from build123d import *

# Parameters (mm, degrees)
SKETCH004_W    = 0.45
SKETCH004_H    = 0.4
PAD_DEPTH      = 3.8
PAD_DEPTH_BACK = 2.2
PAD003_DEPTH   = 0.225
PAD002_DEPTH   = 0.225
SKETCH_W       = 5
SKETCH_H       = 1.8
PAD004_DEPTH   = 4.4
CHAMFER_SIZE   = 0.5
SKETCH005_W    = 2.5
SKETCH005_H    = 4.4
PAD005_DEPTH   = 0.7


with BuildPart() as pad:
    # Sketch004 → Pad (new body, two sides)
    with BuildSketch(Plane.XY) as pad_sk:
        with Locations((1.27, -1.27)):
            Rectangle(SKETCH004_W, SKETCH004_H)
        with Locations((3.81, -1.261698)):
            Rectangle(SKETCH004_W, SKETCH004_H)
    extrude(amount=PAD_DEPTH)
    extrude(pad_sk.sketch, amount=-PAD_DEPTH_BACK)


with BuildPart() as pad003:
    # Sketch003 → Pad003 (new body, symmetric)
    with BuildSketch(Plane(origin=(2.54, -1.27, 0), x_dir=(0, 1, 0), z_dir=(1, 0, 0))):
        Polygon((-0.19, 3.8), (0.19, 3.8), (0.19, 1.6), (1.46, 0.33), (1.46, -2.2), (1.08, -2.2), (1.08, 0.03), (-0.19, 1.3), align=None)
    extrude(amount=PAD003_DEPTH, both=True)


with BuildPart() as pad002:
    # Sketch002 → Pad002 (new body, symmetric)
    with BuildSketch(Plane(origin=(0, -1.27, 0), x_dir=(0, 1, 0), z_dir=(1, 0, 0))):
        Polygon((-0.19, 3.8), (0.19, 3.8), (0.19, 1.6), (1.46, 0.33), (1.46, -2.2), (1.08, -2.2), (1.08, 0.03), (-0.19, 1.3), align=None)
    extrude(amount=PAD002_DEPTH, both=True)


with BuildPart() as sharp_is471f:
    # Sketch → Pad004 (new body)
    with BuildSketch(Plane.XY.offset(3.8)):
        with Locations((1.905, -1.27)):
            Rectangle(SKETCH_W, SKETCH_H)
    extrude(amount=PAD004_DEPTH)

    # Chamfer
    chamfer_edges = [sharp_is471f.edges().sort_by_distance(p)[0] for p in [
        (4.405, -1.27, 8.2),
        (-0.595, -1.27, 8.2),
    ]]
    chamfer(chamfer_edges, length=CHAMFER_SIZE)

    # Sketch005 → Pad005 (new body)
    with BuildSketch(Plane(origin=(0, -0.37, 3.8), x_dir=(-1, 0, 0), z_dir=(0, 1, 0))):
        with Locations((-1.905, 2.2)):
            Rectangle(SKETCH005_W, SKETCH005_H)
    extrude(amount=PAD005_DEPTH)

    add(pad.part)
    add(pad003.part)
    add(pad002.part)


solid = sharp_is471f.part
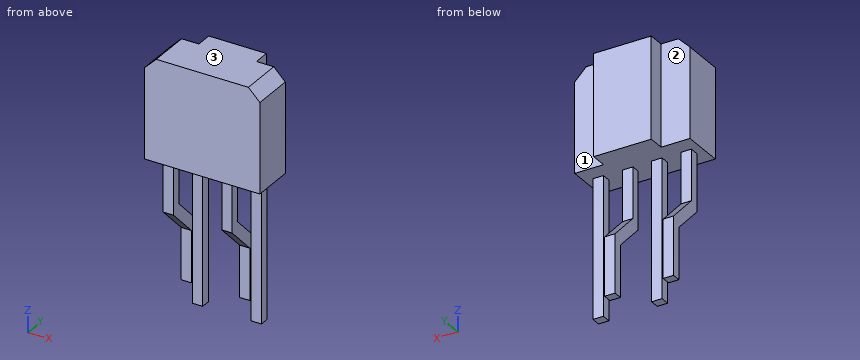
Read the model definition and answer for the solid it produces. Units are mm, in the model's axes. Face numbers are marked on the shaded views. A direction names the side the tool comes from. Coordinates: 2 decimals unless noted, no trailing zeros. Order: outer loops, then holes, each group sorted by start corner. A loop starts at its lowest first (then second) coordinate and runs counter-clockwise, first axis right, second up. Notation, with made-up numbers: M -17.5,68 L 40.5,68 A13 ccw 40.5,91 Z; hole C 0,56.25 d9. An arc over 180 degrees is marked long. Put each result on its own line as item: value. Start each with the question number.
Item 1: For the marked faces 1, 2 and 3, determine the directions among +Z, -Z, +X, -X, +Y, -Y from which every point of the face is accessible in a straight line to the end or side of a thin tool.
Item 2: Section D-D, the plane z = 7.5 is taken. Determine the outline of the cut face in (x, y) (3 decimals), plus the area to 4 significant figures.
Item 3: Section C-C, the plane x = 2.6 is taken. Determine the outline of the cut face in (y, z).
Item 4: Consider probe 1 along Z at (x, y) = (1, -0.15); probe 2 along Y at (x, z) = (-0.2, 6.25); probe 3 along Y at (x, z) = (1.2, 2). Determine where each line is inside the solid, lowest interval first. Write a range as [from, to].
Item 5: Section A-A, the plane z = -0.25 is taken. Determine the outline of the cut face in (x, y) (3 decimals).
Item 6: Given pin 1 Ø0.5 at (x, z) = (4, -0.5) entering from +Y; pin 2 Ø3 at (x, z) = (2.5, 1) entering from -Y; pin 3 Ø0.6 at (y, z) = (0, 5.5) entering from -X (3 decimals), each flat-ended and moving along its own axis, determine where each tip first touches the part or whether it passes through.
Item 7: Section B-B, the plane y = 0 is taken. Determine the outline of the cut face in (x, z) (3 decimals), plus the area to 3 significant figures.
Computed:
1. face 1: +Z, -Z, +X, +Y
1. face 2: +Z, -X, +Y
1. face 3: +Z, +X, -X, +Y, -Y
2. outline: M -0.595,-2.17 L 4.405,-2.17 L 4.405,-0.37 L 3.155,-0.37 L 3.155,0.33 L 0.655,0.33 L 0.655,-0.37 L -0.595,-0.37 Z
2. area: 10.75 mm2
3. outline: M -2.17,3.8 L -1.46,3.8 L -1.46,1.3 L -0.19,0.03 L -0.19,-2.2 L 0.19,-2.2 L 0.19,0.33 L -1.08,1.6 L -1.08,3.8 L 0.33,3.8 L 0.33,8.2 L -2.17,8.2 Z
4. probe 1: z = [3.8, 8.2]
4. probe 2: y = [-2.17, -0.37]
4. probe 3: y = [-1.47, -1.07]
5. outline: M -0.225,-0.19 L 0.225,-0.19 L 0.225,0.19 L -0.225,0.19 Z; M 1.045,-1.47 L 1.495,-1.47 L 1.495,-1.07 L 1.045,-1.07 Z; M 2.315,-0.19 L 2.765,-0.19 L 2.765,0.19 L 2.315,0.19 Z; M 3.585,-1.462 L 4.035,-1.462 L 4.035,-1.062 L 3.585,-1.062 Z
6. pin 1: stops at y = -1.06
6. pin 2: stops at y = -1.47
6. pin 3: stops at x = 0.655
7. outline: M -0.225,-2.2 L 0.225,-2.2 L 0.225,0.52 L -0.225,0.52 Z; M 0.655,3.8 L 3.155,3.8 L 3.155,8.2 L 0.655,8.2 Z; M 2.315,-2.2 L 2.765,-2.2 L 2.765,0.52 L 2.315,0.52 Z
7. area: 13.4 mm2
